```python
from build123d import *

# Parameters (mm, degrees)
F0_R     = 3.8
F1_DEPTH = 1
F2_DEPTH = 10


with BuildPart() as f1:
    # F0 (on Front) → F1 (new body)
    with BuildSketch(Plane.XZ):
        with BuildLine():
            Line((-11.778597, 6.457385), (-15.987552, 0.582385))
            ThreePointArc((-15.987552, 0.582385), (-16.17464, 0), (-15.987552, -0.582385))
            Line((-15.987552, -0.582385), (-11.778597, -6.457385))
            ThreePointArc((-11.778597, -6.457385), (-11.422639, -6.76449), (-10.965684, -6.875))
            Line((-10.965684, -6.875), (10.965684, -6.875))
            ThreePointArc((10.965684, -6.875), (11.422639, -6.76449), (11.778597, -6.457385))
            Line((11.778597, -6.457385), (15.987552, -0.582385))
            ThreePointArc((15.987552, -0.582385), (16.17464, 0), (15.987552, 0.582385))
            Line((15.987552, 0.582385), (11.778597, 6.457385))
            ThreePointArc((11.778597, 6.457385), (11.422639, 6.76449), (10.965684, 6.875))
            Line((10.965684, 6.875), (-10.965684, 6.875))
            ThreePointArc((-10.965684, 6.875), (-11.422639, 6.76449), (-11.778597, 6.457385))
        make_face()
        Circle(F0_R, mode=Mode.SUBTRACT)
    extrude(amount=F1_DEPTH)

    # F0 (on Front) → F2 (join)
    with BuildSketch(Plane.XZ):
        with BuildLine():
            Line((11.736274, 8.375), (-11.736274, 8.375))
            ThreePointArc((-11.736274, 8.375), (-12.193228, 8.26449), (-12.549187, 7.957385))
            Line((-12.549187, 7.957385), (-17.832769, 0.582385))
            ThreePointArc((-17.832769, 0.582385), (-18.019856, 0), (-17.832769, -0.582385))
            Line((-17.832769, -0.582385), (-12.549187, -7.957385))
            ThreePointArc((-12.549187, -7.957385), (-12.193228, -8.26449), (-11.736274, -8.375))
            Line((-11.736274, -8.375), (11.736274, -8.375))
            ThreePointArc((11.736274, -8.375), (12.193228, -8.26449), (12.549187, -7.957385))
            Line((12.549187, -7.957385), (17.832769, -0.582385))
            ThreePointArc((17.832769, -0.582385), (18.019856, 0), (17.832769, 0.582385))
            Line((17.832769, 0.582385), (12.549187, 7.957385))
            ThreePointArc((12.549187, 7.957385), (12.193228, 8.26449), (11.736274, 8.375))
        make_face()
        with BuildLine():
            ThreePointArc((-15.987552, -0.582385), (-16.17464, 0), (-15.987552, 0.582385))
            Line((-15.987552, 0.582385), (-11.778597, 6.457385))
            ThreePointArc((-11.778597, 6.457385), (-11.422639, 6.76449), (-10.965684, 6.875))
            Line((-10.965684, 6.875), (10.965684, 6.875))
            ThreePointArc((10.965684, 6.875), (11.422639, 6.76449), (11.778597, 6.457385))
            Line((11.778597, 6.457385), (15.987552, 0.582385))
            ThreePointArc((15.987552, 0.582385), (16.17464, 0), (15.987552, -0.582385))
            Line((15.987552, -0.582385), (11.778597, -6.457385))
            ThreePointArc((11.778597, -6.457385), (11.422639, -6.76449), (10.965684, -6.875))
            Line((10.965684, -6.875), (-10.965684, -6.875))
            ThreePointArc((-10.965684, -6.875), (-11.422639, -6.76449), (-11.778597, -6.457385))
            Line((-11.778597, -6.457385), (-15.987552, -0.582385))
        make_face(mode=Mode.SUBTRACT)
    extrude(amount=F2_DEPTH)


solid = f1.part
```
For this review, take the finished solid that the model builds, in its own axes (mm). A direction names the side the tool comes from. Coordinates: 2 decimals unless noted, no trailing zeros. Loops run counter-clockwise (first coordinate to the right, second up) from the corner with the lowest first, then second, coordinate; pieces in that order, holes last.
1. Mouldability with a two-part tool opening along Z and no side actions: class faces 1 (the cylindrical face through (-12.187, -4.93, 8.268)), 2 (the flat face through (13.854, -5.437, 3.561)), 3 (the cylindrical face through (18.02, -4.93, -0.01)) as +Z half, -Z half, draft (parallel to the pull), parting line (faces both ways), or undercut.
2. Add section D-D, the plane x = -9. Give the boundary of the cut face in (y, z) (3 decimals), then the cut area to 4 significant figures.
3. Add section C-C, the plane x = 0. Give the boundary of the cut face in (y, z) (3 decimals).
4. Add section A-A, the plane z = 0. Give the boundary of the cut face in (x, y).
5. Add section B-B, the plane y = -6. Give the boundary of the cut face in (x, z) (3 decimals).
6. For line 1 (Z direction, x = 0, y = -0.6) (3 decimals); line 2 (Z direction, x = -9.5, y = -3.5) (3 decimals); line 3 (X direction, y = -1.5, z = -1.25), list the stretches that pass through material, from the lowest coordinate up.
7. Insertion check: P1, Ø2, axis at y = -7, z = -4, coming from the -X side; P2, Ø4.5, axis at x = 0, z = 0, coming from the -Y side. Each pin has a flat end and moves straight along its axis. Give the tip position at first contact, or say it passes through.
8. For faces 4 (the flat face through (-0.1, -10, 7.5)), 5 (the cylindrical face through (-11.43, -5.44, 6.76)), list the 3-axis set-ups (+Z, -Z, +X, -X, +Y, -Y) from which the entire face can be reached by the end or side of a thin tool; tool diameter is ignored.
Result:
1. face 1: +Z half
1. face 2: undercut
1. face 3: parting line
2. outline: (-10, -8.375) - (0, -8.375) - (0, 8.375) - (-10, 8.375) - (-10, 6.875) - (-1, 6.875) - (-1, -6.875) - (-10, -6.875) - close
2. area: 43.75 mm2
3. outline: (-10, -8.375) - (0, -8.375) - (0, -3.8) - (-1, -3.8) - (-1, -6.875) - (-10, -6.875) - close; (-10, 6.875) - (-1, 6.875) - (-1, 3.8) - (0, 3.8) - (0, 8.375) - (-10, 8.375) - close
4. outline: (-18.02, -10) - (-16.17, -10) - (-16.17, -1) - (-3.8, -1) - (-3.8, 0) - (-18.02, 0) - close; (3.8, -1) - (16.17, -1) - (16.17, -10) - (18.02, -10) - (18.02, 0) - (3.8, 0) - close
5. outline: (-17.833, -0.582) - (-12.549, -7.957) arc R1 ccw to (-11.736, -8.375) - (11.736, -8.375) arc R1 ccw to (12.549, -7.957) - (17.833, -0.582) arc R1 ccw to (17.833, 0.582) - (12.549, 7.957) arc R1 ccw to (11.736, 8.375) - (-11.736, 8.375) arc R1 ccw to (-12.549, 7.957) - (-17.833, 0.582) arc R1 ccw to start; hole (-15.988, -0.582) - (-11.779, -6.457) arc R1 ccw to (-10.966, -6.875) - (10.966, -6.875) arc R1 ccw to (11.779, -6.457) - (15.988, -0.582) arc R1 ccw to (15.988, 0.582) - (11.779, 6.457) arc R1 ccw to (10.966, 6.875) - (-10.966, 6.875) arc R1 ccw to (-11.779, 6.457) - (-15.988, 0.582) arc R1 ccw to start
6. line 1: z = -8.375 to -3.8, 3.8 to 8.375
6. line 2: z = -8.375 to -6.875, 6.875 to 8.375
6. line 3: x = -17.35 to -15.51, 15.51 to 17.35
7. P1: stops at x = -16.1
7. P2: passes through
8. face 4: +Z, -Z, +X, -X, -Y
8. face 5: -Y
